The listing builds one solid part. Answer for the finished solid, in the listing's coordinates (mm). Give positions to 0.01 mm unless a question says otherwise; leave off trailing zeros. Loops run counter-clockwise (first coordinate to the right, second up) from the corner with the lowest first, then second, coordinate; pieces in that order, holes last.
Item 1: Section A-A, the plane z = 0 is taken. Give the vertices of the cut face in (x, y) (3 decimals).
Item 2: Consider line 1 along X through (y, z) = (2.25, 0); line 2 along X through (y, z) = (1.5, 11); line 3 along X through (y, z) = (3, 17). Determine where each line is inside the solid, lowest interval first.
Item 3: Section C-C, the plane z = 39 is taken. Give the vertices of the cut face in (x, y) (3 decimals).
Item 4: Each of these flat-tipped pins is pushed along its axis until it touches: pin 1 Ø2.5 at (x, z) = (0, -33.02) entering from -Y; pin 2 Ø1.5 at (x, y) = (21.5, 4) entering from -Z. Where does it stop, or does it pass through?
Item 5: Section B-B, the plane x = 33.02 is taken. Give the vertices of the cut face in (y, z) (3 decimals).
Item 6: Section D-D, the plane y = 3 is taken. Give the vertices of the cut face in (x, z) (1 decimal), and give its area (3 significant figures).
from build123d import *

# Parameters (mm, degrees)
SKETCH1_R           = 75
BOSS_EXTRUDE1_DEPTH = 9.525
CUT_EXTRUDE2_REACH  = 108.493
FILLET1_R           = 10.16
SKETCH39_R          = 22.86
SKETCH39_R_2        = 2.0193
CUT_EXTRUDE30_DEPTH = 247.31360274
SKETCH42_R          = 2.0193
CUT_EXTRUDE33_DEPTH = 247.31360274
CUT_EXTRUDE35_DEPTH = 247.31360274


with BuildPart() as part:
    # Sketch1 → Boss-Extrude1 (new body)
    with BuildSketch(Plane(origin=(0, 0, 0), x_dir=(1, 0, 0), z_dir=(0, 1, 0))):
        with Locations(Location((0, 0, 0), (0, 0, 90))):
            Circle(SKETCH1_R)
    extrude(amount=BOSS_EXTRUDE1_DEPTH)

    # Sketch11 → Cut-Extrude2 (cut, up to next)
    with BuildSketch(Plane(origin=(0, 9.525, 0), x_dir=(1, 0, 0), z_dir=(0, 1, 0)), mode=Mode.PRIVATE) as cut_extrude2_sk1:
        with BuildLine():
            Line((-54.798637954, 51.206535505), (-32.347997651, 28.755895202))
            ThreePointArc((-32.347997651, 28.755895202), (-28.755895202, 28.755895202), (-28.755895202, 32.347997651))
            Line((-28.755895202, 32.347997651), (-51.206535505, 54.798637954))
            ThreePointArc((-51.206535505, 54.798637954), (-53.033008589, 53.033008589), (-54.798637954, 51.206535505))
        make_face()
    cut_extrude2_tool1 = extrude(cut_extrude2_sk1.sketch, amount=-CUT_EXTRUDE2_REACH, mode=Mode.PRIVATE) & part.part
    # Sketch11 → Cut-Extrude2 (cut, up to next)
    with BuildSketch(Plane(origin=(0, 9.525, 0), x_dir=(1, 0, 0), z_dir=(0, 1, 0)), mode=Mode.PRIVATE) as cut_extrude2_sk2:
        with BuildLine():
            Line((-51.206535505, -54.798637954), (-28.755895202, -32.347997651))
            ThreePointArc((-28.755895202, -32.347997651), (-28.755895202, -28.755895202), (-32.347997651, -28.755895202))
            Line((-32.347997651, -28.755895202), (-54.798637954, -51.206535505))
            ThreePointArc((-54.798637954, -51.206535505), (-53.033008589, -53.033008589), (-51.206535505, -54.798637954))
        make_face()
    cut_extrude2_tool2 = extrude(cut_extrude2_sk2.sketch, amount=-CUT_EXTRUDE2_REACH, mode=Mode.PRIVATE) & part.part
    add(cut_extrude2_tool1.solids().sort_by_distance((-41.078737, 9.525, -41.078737))[0], mode=Mode.SUBTRACT)
    add(cut_extrude2_tool2.solids().sort_by_distance((-41.078737, 9.525, 41.078737))[0], mode=Mode.SUBTRACT)

    # Fillet1
    fillet1_edges = [part.edges().sort_by_distance(p)[0] for p in [
        (-51.206535505, 4.7625, 54.798637954),
        (-54.798637954, 4.7625, 51.206535505),
        (-54.798637954, 4.7625, -51.206535505),
        (-51.206535505, 4.7625, -54.798637954),
    ]]
    fillet(fillet1_edges, radius=FILLET1_R)

    # Sketch39 → Cut-Extrude30 (cut, through all)
    with BuildSketch(Plane(origin=(-73.768816189, 9.525, -121.080352405), x_dir=(1, 0, 0), z_dir=(0, 1, 0))):
        with Locations(Location((73.768816189, -121.080352405, 0), (0, 0, 270))):
            Circle(SKETCH39_R)
        with Locations(Location((73.768816189, -88.060352405, 0), (0, 0, 270))):
            Circle(SKETCH39_R_2)
        with Locations(Location((106.788816189, -121.080352405, 0), (0, 0, 270))):
            Circle(SKETCH39_R_2)
        with Locations(Location((73.768816189, -154.100352405, 0), (0, 0, 270))):
            Circle(SKETCH39_R_2)
        with Locations(Location((40.748816189, -121.080352405, 0), (0, 0, 270))):
            Circle(SKETCH39_R_2)
    extrude(amount=-CUT_EXTRUDE30_DEPTH, mode=Mode.SUBTRACT)

    # Sketch42 → Cut-Extrude33 (cut, through all)
    with BuildSketch(Plane(origin=(-73.768816189, 9.525, -121.080352405), x_dir=(1, 0, 0), z_dir=(0, 1, 0))):
        with Locations(Location((48.605023435, -95.916559651, 0), (0, 0, 270))):
            Circle(SKETCH42_R)
    extrude(amount=-CUT_EXTRUDE33_DEPTH, mode=Mode.SUBTRACT)

    # Sketch44 → Cut-Extrude35 (cut, through all)
    with BuildSketch(Plane(origin=(-73.768816189, 9.525, -121.080352405), x_dir=(1, 0, 0), z_dir=(0, 1, 0))):
        with BuildLine():
            ThreePointArc((34.405967979, -136.122213123), (36.00963526, -139.786919397), (37.953573181, -143.283049568))
            ThreePointArc((37.953573181, -143.283049568), (46.974494303, -145.399596657), (49.091041391, -136.378675534))
            ThreePointArc((49.091041391, -136.378675534), (47.751609959, -133.969737166), (46.646635186, -131.444644817))
            ThreePointArc((46.646635186, -131.444644817), (38.18751743, -127.663095366), (34.405967979, -136.122213123))
        make_face()
    extrude(amount=-CUT_EXTRUDE35_DEPTH, mode=Mode.SUBTRACT)


solid = part.part
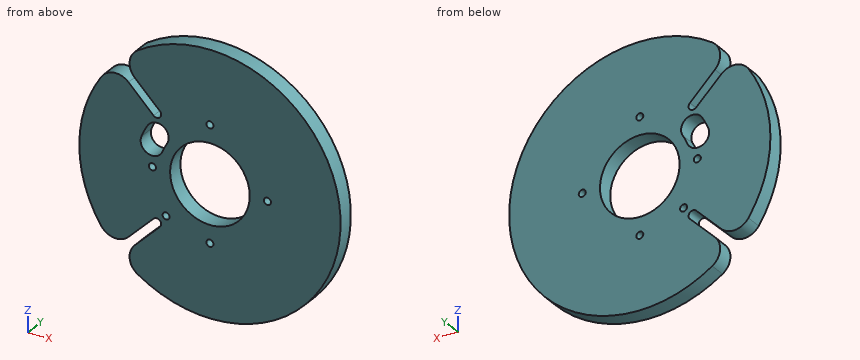
Worked answers:
1. outline: (-75, 0) - (-35.039, 0) - (-35.039, 9.525) - (-75, 9.525) - close; (-31.001, 0) - (-22.86, 0) - (-22.86, 9.525) - (-31.001, 9.525) - close; (22.86, 0) - (31.001, 0) - (31.001, 9.525) - (22.86, 9.525) - close; (35.039, 0) - (75, 0) - (75, 9.525) - (35.039, 9.525) - close
2. line 1: x = -75 to -35.04, -31 to -22.86, 22.86 to 31, 35.04 to 75
2. line 2: x = -74.19 to -39.57, -26.87 to -20.04, 20.04 to 74.19
2. line 3: x = -73.05 to -38.56, -23.93 to -15.28, 15.28 to 73.05
3. outline: (-64.062, 0) - (-42.592, 0) - (-42.592, 9.525) - (-64.062, 9.525) - close; (-35.408, 0) - (64.062, 0) - (64.062, 9.525) - (-35.408, 9.525) - close
4. pin 1: passes through
4. pin 2: stops at z = -72.07
5. outline: (0, -67.34) - (9.525, -67.34) - (9.525, -2.019) - (0, -2.019) - close; (0, 2.019) - (9.525, 2.019) - (9.525, 67.34) - (0, 67.34) - close
6. outline: (-62.4, -41.6) arc R10.2 ccw to (-46.8, -43.2) - (-32.3, -28.8) arc R2.5 cw to (-28.8, -32.3) - (-43.2, -46.8) arc R10.2 ccw to (-41.6, -62.4) arc R75 ccw (long way) to (-41.6, 62.4) arc R10.2 ccw to (-43.2, 46.8) - (-28.8, 32.3) arc R2.5 cw to (-32.3, 28.8) - (-46.8, 43.2) arc R10.2 ccw to (-62.4, 41.6) arc R75 ccw to start; hole (-39.4, 15) arc R6.6 ccw to (-27.1, 10.4) arc R29 cw to (-24.7, 15.3) arc R6.6 ccw to (-35.8, 22.2) arc R42.1 ccw to start; hole circle Ø4 at (-33, 0); hole circle Ø4 at (-25.2, -25.2); hole circle Ø45.7 at (0, 0); hole circle Ø4 at (0, -33); hole circle Ø4 at (0, 33); hole circle Ø4 at (33, 0)
6. area: 15,300 mm2
